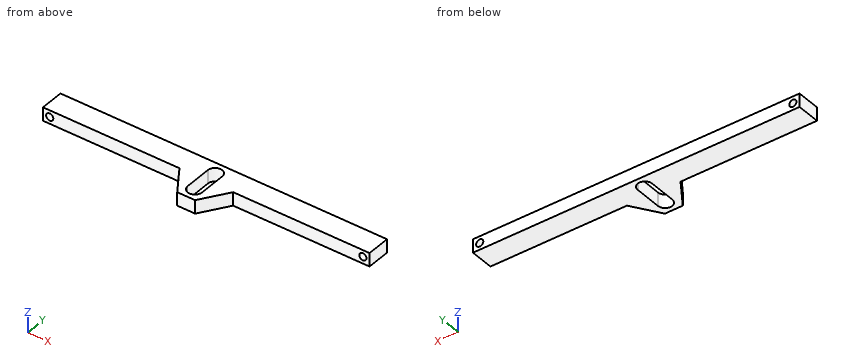
from build123d import *

# Parameters (mm, degrees)
BOSS_EXTRUDE1_DEPTH = 3
SKETCH2_R           = 0.8
CUT_EXTRUDE1_DEPTH  = 50.180347904


with BuildPart() as part:
    # Sketch1 → Boss-Extrude1 (new body)
    with BuildSketch(Plane.XY):
        Polygon((-48.720700118, 1.790980695), (-18.220700118, 1.790980695), (-14.220700118, -4.209019305), (-10.220700118, -4.209019305), (-6.220700118, 1.790980695), (24.279299882, 1.790980695), (24.279299882, 6.990980695), (-48.720700118, 6.990980695), align=None)
        with BuildLine():
            ThreePointArc((-10.620700118, -1.609019305), (-12.220700118, -3.209019305), (-13.820700118, -1.609019305))
            Line((-13.820700118, -1.609019305), (-13.820700118, 4.390980695))
            ThreePointArc((-13.820700118, 4.390980695), (-12.220700118, 5.990980695), (-10.620700118, 4.390980695))
            Line((-10.620700118, 4.390980695), (-10.620700118, -1.609019305))
        make_face(mode=Mode.SUBTRACT)
    extrude(amount=BOSS_EXTRUDE1_DEPTH)

    # Sketch2 → Cut-Extrude1 (cut, through all)
    with BuildSketch(Plane.XZ.offset(-1.790980695)):
        with Locations(Location((22.779299882, 1.5, 0), (0, 0, 270))):
            Circle(SKETCH2_R)
        with Locations(Location((-47.220700118, 1.5, 0), (0, 0, 270))):
            Circle(SKETCH2_R)
    extrude(amount=-CUT_EXTRUDE1_DEPTH, mode=Mode.SUBTRACT)


solid = part.part
Design review of the part built by this model. Coordinates are the model's own, in mm. Coordinates: 2 decimals unless noted, no trailing zeros. Order: outer loops, then holes, each group sorted by start corner. A loop starts at its lowest first (then second) coordinate and runs counter-clockwise, first axis right, second up. Notation, with made-up numbers: (-35, 36.5) -> (-18, 36.5) arc R25 ccw to (-18, 65.5) -> close; hole circle Ø1 at (-23, -24). An arc over 180 degrees is marked (long way). Use one line per item in the form item = value. Start each with the question number.
(1) Add section B-B on y = 0.75. State the section outline as (x, z) points.
(2) Add section D-D on y = 5.25. State the section outline as (x, z) points, plus the area to 3 significant figures.
(3) Add section A-A on z = 1.5. State the section outline as (x, y) points, plus the area to 3 significant figures.
(4) Insertion check: pin 1 (3 mm diameter, centred on x = 10.5, y = -1, fed in from +Z) (3 decimals); pin 2 (1.5 mm diameter, centred on y = 0.5, z = 2, fed in from +X); pin 3 (1.5 mm diameter, centred on x = -29, z = 1, fed in from -Y); pin 4 (1.5 mm diameter, centred on y = -2.5, z = 0.5, fed in from +X). Each pin has a flat end and moves straight along its axis. Give the tip position at first contact, or say it passes through.
(5) For probe 1 along X at (y, z) = (6.5, 1.4); probe 2 along X at (y, z) = (3.6, 1.5); probe 3 along X at (y, z) = (3.5, 2.65), list the stretches that pass through material, from the lowest coordinate up.
(6) Add section C-C on x = -12.5. State the section outline as (y, z) points, plus the area to 3 significant figures.
Answer block:
q1.outline = (-17.53, 0) -> (-13.82, 0) -> (-13.82, 3) -> (-17.53, 3) -> close; (-10.62, 0) -> (-6.91, 0) -> (-6.91, 3) -> (-10.62, 3) -> close
q2.outline = (-48.72, 0) -> (-13.57, 0) -> (-13.57, 3) -> (-48.72, 3) -> close; (-10.87, 0) -> (24.28, 0) -> (24.28, 3) -> (-10.87, 3) -> close; hole circle Ø1.6 at (-47.22, 1.5); hole circle Ø1.6 at (22.78, 1.5)
q2.area = 207 mm²
q3.outline = (-48.72, 1.79) -> (-48.02, 1.79) -> (-48.02, 6.99) -> (-48.72, 6.99) -> close; (-46.42, 1.79) -> (-18.22, 1.79) -> (-14.22, -4.21) -> (-10.22, -4.21) -> (-6.22, 1.79) -> (21.98, 1.79) -> (21.98, 6.99) -> (-46.42, 6.99) -> close; (23.58, 1.79) -> (24.28, 1.79) -> (24.28, 6.99) -> (23.58, 6.99) -> close; hole (-13.82, -1.61) arc R1.6 ccw to (-10.62, -1.61) -> (-10.62, 4.39) arc R1.6 ccw to (-13.82, 4.39) -> close
q3.area = 384 mm²
q4.pin_1 = through
q4.pin_2 = -6.58
q4.pin_3 = 1.79
q4.pin_4 = -8.58
q5.probe_1 = -48.72 to -48.01, -46.43 to 21.99, 23.57 to 24.28
q5.probe_2 = -48.72 to -48.02, -46.42 to -13.82, -10.62 to 21.98, 23.58 to 24.28
q5.probe_3 = -48.72 to -13.82, -10.62 to 24.28
q6.outline = (-4.21, 0) -> (-3.18, 0) -> (-3.18, 3) -> (-4.21, 3) -> close; (5.97, 0) -> (6.99, 0) -> (6.99, 3) -> (5.97, 3) -> close
q6.area = 6.15 mm²
